from build123d import *

# Parameters (mm, degrees)
SKETCH7_R           = 317.5
CUT_EXTRUDE2_DEPTH  = 88.9
SKETCH8_R           = 73.025
SKETCH8_R_2         = 69.85
BOSS_EXTRUDE1_DEPTH = 76.2


with BuildPart() as part:
    # Sketch2 → Revolve1 (revolve)
    with BuildSketch(Plane.XY):
        with BuildLine():
            Line((-76.2, 0), (-69.85, 0))
            ThreePointArc((-69.85, 0), (-46.178344337, 164.977710697), (0, 325.12))
            Line((0, 325.12), (0, 330.2))
            ThreePointArc((0, 330.2), (-50.970594074, 168.070137094), (-76.2, 0))
        make_face()
    revolve(axis=Axis((0, 330.2, 0), (0, -1, 0)))

    # Sketch7 → Cut-Extrude2 (cut)
    with BuildSketch(Plane(origin=(0, 381, 0), x_dir=(1, 0, 0), z_dir=(0, 1, 0))):
        Circle(SKETCH7_R)
    extrude(amount=-CUT_EXTRUDE2_DEPTH, mode=Mode.SUBTRACT)

    # Sketch8 → Boss-Extrude1 (add)
    with BuildSketch(Plane.XZ):
        Circle(SKETCH8_R)
        Circle(SKETCH8_R_2, mode=Mode.SUBTRACT)
    extrude(amount=BOSS_EXTRUDE1_DEPTH)


solid = part.part
Design review of the part built by this model. Coordinates are the model's own, in mm. Round coordinates to 2 decimals unless told otherwise and drop trailing zeros. Loops run counter-clockwise (first coordinate to the right, second up) from the corner with the lowest first, then second, coordinate; pieces in that order, holes last. Notation, with made-up numbers: (-24, 88.5) - (18, 88.5) arc R13 cw to (18, 104.5) - close; hole circle Ø9 at (71.5, -28). An arc over 180 degrees is marked (long way). One line per item, written item: value. Start each with the question number.
1) Draft analysis for pull direction Z (two halves, no side actions). For faces 1 (the cylindrical face through (-55.431, -37.567, -42.503)), 2 (the cylindrical face through (69.653, -37.567, 21.935)), 3 (the flat face through (-62, 0, 39)), state which applies: +Z half, -Z half, draft (parallel to the pull), parting line (faces both ways), or undercut.
2) Insertion check: pin 1 Ø5 at (x, y) = (-49.5, -21) entering from -Z; pin 2 Ø8 at (y, z) = (78.5, 51.5) entering from -X; pin 3 Ø10 at (x, y) = (29, 189) entering from +Z. Each pin has a flat end and moves straight along its axis. Give the tip position at first contact, or say it passes through.
3) Consider section A-A on y = -4.5. Give the boundary of the cut face in (x, z) (3 decimals), then the cut area to 3 significant figures.
4) To check wall thickness, follow L1, parallel to Z at x = 0, y = -31 (3 decimals); L2, parallel to X at y = -30, z = 12; L3, parallel to X at y = 90.5, z = -33.5. State the ranges of each line that lie inside material, in increasing order. Write a range as from..to.
Reported:
1. face 1: undercut
1. face 2: parting line
1. face 3: draft
2. pin 1: stops at z = -55.89
2. pin 2: stops at x = -48.38
2. pin 3: stops at z = 39.49
3. outline: circle Ø146.05 at (0, 0); hole circle Ø139.7 at (0, 0)
3. area: 1,430 mm^2
4. L1: z = -73.025..-69.85, 69.85..73.025
4. L2: x = -72.03..-68.81, 68.81..72.03
4. L3: x = -56.8..-49.48, 49.48..56.8
